Model file for the job. Use its own axes, mm. Face numbers are marked on the shaded views. A direction names the side the tool comes from. Coordinates: 2 decimals unless noted, no trailing zeros. Write each loop counter-clockwise with the first axis right and the second up, starting at its lowest first coordinate (ties: lowest second). Pieces come first, ordered by that corner, then holes. Notation, with made-up numbers: M 57.25,57 L 108.25,57 A12 ccw 108.25,80 Z; hole C 58.25,44.25 d2. An arc over 180 degrees is marked long. Put each result on its own line as item: value. Start each with the question number.
Q1. Cut at C-C (z = 17). Write the cut outline in (x, y), then the cut area to 3 significant figures.
Q2. Cut at B-B (y = -29). Write the cut outline in (x, z) (3 decimals), then the cut area to 3 significant figures.
Q3. Which spindle directions (+Z, -Z, +X, -X, +Y, -Y) get a long thin tool onto all of the face, cutting with end or side? Do the marked faces 1, 2, 3 and 4. Say none if no direction does.
Q4. Drop flat-ended pins along their axis: pin 1 (4 mm diameter, centred on y = -16, z = 12.5, fed in from -X); pin 2 (1 mm diameter, centred on y = -17.5, z = -7, fed in from -X); pin 3 (9.5 mm diameter, centred on x = 29, y = -5.5, fed in from -Z) (3 decimals). Give the stop position or say it passes through.
Q5. Drill centre lines: line 1 along Z through (x, y) = (6, -29); line 2 along Y through (x, z) = (36, 11); line 3 along Y through (x, z) = (38, 0.5). Where is each one in solid material? Low to high.
Q6. Cut at D-D (x = 3.5). Write the cut outline in (y, z).
Q7. Cut at A-A (x = 32.5). Write the cut outline in (y, z) (3 decimals).
Q8. Pull direction Y, two halves, no side cores. Call the marked faces 5, 6, 7 and 8: pulls with the +Y half, pulls with the -Y half, needs draft (parallel to the pull), parting line crosses it, or undercut.
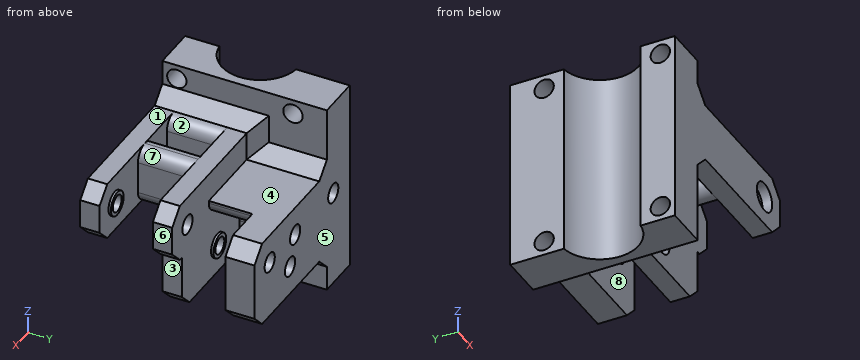
```python
from build123d import *

# Parameters (mm, degrees)
BOSS_EXTRUDE1_DEPTH      = 20
BOSS_EXTRUDE1_DEPTH_BACK = 20
SKETCH2_R                = 1.75
CUT_EXTRUDE1_DEPTH       = 59.72818744
SKETCH3_R                = 2
CUT_EXTRUDE2_DEPTH       = 7
CUT_EXTRUDE3_REACH       = 60.728
CUT_EXTRUDE4_REACH       = 54.783
CUT_EXTRUDE5_REACH       = 58.648
BOSS_EXTRUDE3_DEPTH      = 9
SKETCH10_W               = 5.38
SKETCH10_H               = 12
SKETCH10_W_2             = 5.81
BOSS_EXTRUDE4_DEPTH      = 11
FILLET1_R                = 2.69
FILLET2_R                = 2.69
FILLET3_R                = 2.69
CHAMFER1_SIZE            = 3
CUT_EXTRUDE8_REACH       = 51.774
SKETCH14_R               = 2
SKETCH16_R               = 2
CUT_EXTRUDE9_DEPTH       = 10
BOSS_EXTRUDE5_START      = 0.5
SKETCH17_R               = 2.5
SKETCH17_R_2             = 1.75
BOSS_EXTRUDE5_DEPTH      = 0.5
BOSS_EXTRUDE6_START      = 0.5
SKETCH18_R               = 2.5
SKETCH18_R_2             = 1.75
BOSS_EXTRUDE6_DEPTH      = 0.5
SKETCH20_R               = 3
CUT_EXTRUDE10_DEPTH      = 2
SKETCH21_R               = 3
CUT_EXTRUDE11_DEPTH      = 2
SKETCH11_R               = 2
CUT_EXTRUDE6_DEPTH       = 10
SKETCH12_W               = 1
SKETCH12_H               = 32
CUT_EXTRUDE7_DEPTH       = 67.426230512
BOSS_EXTRUDE7_DEPTH      = 4
BOSS_EXTRUDE8_START      = 2
SKETCH23_R               = 2
BOSS_EXTRUDE8_DEPTH      = 2


# Some blends are built 0.0001 mm under size
with BuildPart() as part:
    # Sketch1 → Boss-Extrude1 (new, two sides: drawn at the far end of the back side and taken through both)
    with BuildSketch(Plane.XY.offset(-BOSS_EXTRUDE1_DEPTH_BACK)):
        with BuildLine():
            Line((0, 0), (45, 0))
            Line((45, 0), (45, -4))
            Line((45, -4), (10, -4))
            Line((10, -4), (10, -13))
            Line((10, -13), (45, -13))
            Line((45, -13), (45, -17))
            Line((45, -17), (10, -17))
            Line((10, -17), (10, -28))
            Line((10, -28), (45, -28))
            Line((45, -28), (45, -32))
            Line((45, -32), (0, -32))
            Line((0, -32), (0, -28))
            Line((0, -28), (0, -25))
            ThreePointArc((0, -25), (8, -17), (0, -9))
            Line((0, -9), (0, -4))
            Line((0, -4), (0, 0))
        make_face()
    extrude(amount=BOSS_EXTRUDE1_DEPTH + BOSS_EXTRUDE1_DEPTH_BACK)

    # Sketch2 → Cut-Extrude1 (cut, through all)
    with BuildSketch(Plane(origin=(0, 0, 0), x_dir=(1, 0, 0), z_dir=(0, 1, 0))):
        with Locations(Location((24.5, 5.895, 0), (0, 0, 270))):
            Circle(SKETCH2_R)
        with Locations(Location((36.29, -5.895, 0), (0, 0, 270))):
            Circle(SKETCH2_R)
    extrude(amount=-CUT_EXTRUDE1_DEPTH, mode=Mode.SUBTRACT)

    # Sketch3 → Cut-Extrude2 (cut)
    with BuildSketch(Plane(origin=(0, 0, 0), x_dir=(1, 0, 0), z_dir=(0, 1, 0))):
        with Locations(Location((7.5, 0, 0), (0, 0, 270))):
            Circle(SKETCH3_R)
        with Locations(Location((22.5, 0, 0), (0, 0, 270))):
            Circle(SKETCH3_R)
        with Locations(Location((32.5, 0, 0), (0, 0, 270))):
            Circle(SKETCH3_R)
    extrude(amount=-CUT_EXTRUDE2_DEPTH, mode=Mode.SUBTRACT)

    # Sketch5 → Cut-Extrude3 (cut, up to next)
    with BuildSketch(Plane(origin=(0, 0, 0), x_dir=(1, 0, 0), z_dir=(0, 1, 0)), mode=Mode.PRIVATE) as cut_extrude3_sk1:
        Polygon((10, 20), (10, 11.895), (35.5, 11.895), (38.5, 8.895), (38.5, -3), (35.5, -6), (10, -6), (10, -20), (45, -20), (45, 20), align=None)
    cut_extrude3_tool1 = extrude(cut_extrude3_sk1.sketch, amount=-CUT_EXTRUDE3_REACH, mode=Mode.PRIVATE) & part.part
    add(cut_extrude3_tool1.solids().sort_by_distance((10.531507, 0, -15.9475))[0], mode=Mode.SUBTRACT)

    # Sketch6 → Cut-Extrude4 (cut, up to next)
    with BuildSketch(Plane(origin=(0, -13, 0), x_dir=(1, 0, 0), z_dir=(0, 1, 0)), mode=Mode.PRIVATE) as cut_extrude4_sk1:
        Polygon((45, 20), (10, 20), (10, 11.895), (35.5, 11.895), (38.5, 8.895), (38.5, 0.105), (39.29, 0.105), (42.29, -2.895), (42.29, -8.895), (39.29, -11.895), (10, -11.895), (10, -20), (45, -20), align=None)
    cut_extrude4_tool1 = extrude(cut_extrude4_sk1.sketch, amount=-CUT_EXTRUDE4_REACH, mode=Mode.PRIVATE) & part.part
    add(cut_extrude4_tool1.solids().sort_by_distance((27.5, -13, -19.468493))[0], mode=Mode.SUBTRACT)

    # Sketch7 → Cut-Extrude5 (cut, up to next)
    with BuildSketch(Plane(origin=(0, -28, 0), x_dir=(1, 0, 0), z_dir=(0, 1, 0)), mode=Mode.PRIVATE) as cut_extrude5_sk1:
        Polygon((10, -11.895), (39.29, -11.895), (42.29, -8.895), (42.29, -2.895), (39.29, 0.105), (10, 0.105), (10, 20), (45, 20), (45, -20), (10, -20), align=None)
    cut_extrude5_tool1 = extrude(cut_extrude5_sk1.sketch, amount=-CUT_EXTRUDE5_REACH, mode=Mode.PRIVATE) & part.part
    add(cut_extrude5_tool1.solids().sort_by_distance((28.13547, -28, -2.184137))[0], mode=Mode.SUBTRACT)

    # Sketch9 → Boss-Extrude3 (add)
    with BuildSketch(Plane(origin=(0, -13, 0), x_dir=(1, 0, 0), z_dir=(0, 1, 0))):
        with BuildLine():
            ThreePointArc((24.5, -2.795), (18.355242071, -0.249757929), (15.81, 5.895))
            Line((15.81, 5.895), (15.81, 11.895))
            Line((15.81, 11.895), (10, 11.895))
            Line((10, 11.895), (10, -6))
            Line((10, -6), (27.895, -6))
            Line((27.895, -6), (27.895, -2.795))
            Line((27.895, -2.795), (24.5, -2.795))
        make_face()
    extrude(amount=BOSS_EXTRUDE3_DEPTH)

    # Sketch10 → Boss-Extrude4 (add)
    with BuildSketch(Plane(origin=(0, -28, 0), x_dir=(1, 0, 0), z_dir=(0, 1, 0))):
        with Locations((24.5, -5.895)):
            Rectangle(SKETCH10_W, SKETCH10_H)
        with Locations((12.905, -5.895)):
            Rectangle(SKETCH10_W_2, SKETCH10_H)
    extrude(amount=BOSS_EXTRUDE4_DEPTH)

    # Fillet1
    # the kernel refuses this fillet: 2.69 mm, written as the material it adds along each edge
    # the kernel refuses this fillet: 2.69 mm, written as the material it takes off along each edge
    with BuildSketch(Plane(origin=(21.81, -28, -0.105), x_dir=(0, 0, 1), z_dir=(0, 1, 0))) as fillet1_2_piece_1:
        with BuildLine():
            CenterArc((FILLET1_R, FILLET1_R), FILLET1_R, 180, 90)
            Line((0, FILLET1_R), (0, 0))
            Line((0, 0), (FILLET1_R, 0))
        make_face()
    extrude(amount=11, mode=Mode.SUBTRACT)
    with BuildSketch(Plane(origin=(27.19, -28, -0.105), x_dir=(0, 0, 1), z_dir=(0, 1, 0))) as fillet1_2_piece_2:
        with BuildLine():
            CenterArc((FILLET1_R, -FILLET1_R), FILLET1_R, 90, 90)
            Line((0, -FILLET1_R), (0, 0))
            Line((0, 0), (FILLET1_R, 0))
        make_face()
    extrude(amount=11, mode=Mode.SUBTRACT)

    # Fillet2
    fillet2_edges = [part.edges().sort_by_distance(p)[0] for p in [
        (27.19, -22.5, 11.895),
        (21.81, -22.5, 11.895),
    ]]
    fillet(fillet2_edges, radius=FILLET2_R - 0.0001)  # a hair under: the kernel refuses the full size

    # Fillet3
    fillet3_edges = [part.edges().sort_by_distance(p)[0] for p in [
        (15.81, -8.5, -11.895),
        (27.895, -8.5, 2.795),
        (15.81, -22.5, -0.105),
        (15.81, -22.5, 11.895),
    ]]
    fillet(fillet3_edges, radius=FILLET3_R)

    # Chamfer1
    chamfer1_edges = [part.edges().sort_by_distance(p)[0] for p in [
        (10, -8.5, -11.895),
        (10, -6.5, 6),
        (10, -17, -6),
        (10, -22.5, 11.895),
        (10, -24.5, -0.105),
        (10, -13, 8.9475),
    ]]
    chamfer(chamfer1_edges, length=CHAMFER1_SIZE)

    # Sketch14 → Cut-Extrude8 (cut, up to next)
    with BuildSketch(Plane.XZ.offset(17), mode=Mode.PRIVATE) as cut_extrude8_sk1:
        with Locations(Location((36.29, 5.895, 0), (0, 0, 270))):
            Circle(SKETCH14_R)
    cut_extrude8_tool1 = extrude(cut_extrude8_sk1.sketch, amount=-CUT_EXTRUDE8_REACH, mode=Mode.PRIVATE) & part.part
    add(cut_extrude8_tool1.solids().sort_by_distance((36.29, -17, 5.895))[0], mode=Mode.SUBTRACT)

    # Sketch16 → Cut-Extrude9 (cut)
    with BuildSketch(Plane.XZ.offset(4)):
        with Locations((24.5, -5.895)):
            Circle(SKETCH16_R)
    extrude(amount=-CUT_EXTRUDE9_DEPTH, mode=Mode.SUBTRACT)

    # Sketch17 → Boss-Extrude5 (add)
    with BuildSketch(Plane(origin=(0, -13, 0), x_dir=(1, 0, 0), z_dir=(0, 1, 0)).offset(BOSS_EXTRUDE5_START)):
        with Locations(Location((24.5, 5.895, 0), (0, 0, 270))):
            Circle(SKETCH17_R)
        with Locations(Location((24.5, 5.895, 0), (0, 0, 270))):
            Circle(SKETCH17_R_2, mode=Mode.SUBTRACT)
    extrude(amount=-BOSS_EXTRUDE5_DEPTH)

    # Sketch18 → Boss-Extrude6 (add)
    with BuildSketch(Plane(origin=(0, -28, 0), x_dir=(1, 0, 0), z_dir=(0, 1, 0)).offset(BOSS_EXTRUDE6_START)):
        with Locations(Location((36.29, -5.895, 0), (0, 0, 270))):
            Circle(SKETCH18_R)
        with Locations(Location((36.29, -5.895, 0), (0, 0, 270))):
            Circle(SKETCH18_R_2, mode=Mode.SUBTRACT)
    extrude(amount=-BOSS_EXTRUDE6_DEPTH)

    # Sketch20 → Cut-Extrude10 (cut)
    with BuildSketch(Plane.XZ.offset(32)):
        with Locations(Location((36.29, 5.895, 0), (0, 0, 270))):
            Circle(SKETCH20_R)
    extrude(amount=-CUT_EXTRUDE10_DEPTH, mode=Mode.SUBTRACT)

    # Sketch21 → Cut-Extrude11 (cut)
    with BuildSketch(Plane.XZ.offset(17)):
        with Locations(Location((24.5, -5.895, 0), (0, 0, 270))):
            Circle(SKETCH21_R)
    extrude(amount=-CUT_EXTRUDE11_DEPTH, mode=Mode.SUBTRACT)

    # Sketch11 → Cut-Extrude6 (cut)
    with BuildSketch(Plane.ZY):
        with Locations(Location((17, -5, 0), (0, 0, 270))):
            Circle(SKETCH11_R)
        with Locations(Location((17, -29, 0), (0, 0, 270))):
            Circle(SKETCH11_R)
        with Locations(Location((-17, -29, 0), (0, 0, 270))):
            Circle(SKETCH11_R)
        with Locations(Location((-17, -5, 0), (0, 0, 270))):
            Circle(SKETCH11_R)
    extrude(amount=-CUT_EXTRUDE6_DEPTH, mode=Mode.SUBTRACT)

    # Sketch12 → Cut-Extrude7 (cut, through all)
    with BuildSketch(Plane.XY.offset(20)):
        with Locations((0.5, -16)):
            Rectangle(SKETCH12_W, SKETCH12_H)
    extrude(amount=-CUT_EXTRUDE7_DEPTH, mode=Mode.SUBTRACT)

    # Sketch22 → Boss-Extrude7 (add)
    with BuildSketch(Plane(origin=(0, 0, 0), x_dir=(1, 0, 0), z_dir=(0, 1, 0))):
        with BuildLine():
            Line((37.136593667, -4.363406333), (35.5, -6))
            Line((35.5, -6), (34.54315284, -6))
            ThreePointArc((34.54315284, -6), (35.356070776, -4.415041823), (37.136593667, -4.363406333))
        make_face()
    extrude(amount=-BOSS_EXTRUDE7_DEPTH)

    # Sketch23 → Boss-Extrude8 (add)
    with BuildSketch(Plane(origin=(0, 0, 0), x_dir=(1, 0, 0), z_dir=(0, 1, 0)).offset(BOSS_EXTRUDE8_START)):
        Polygon((35.5, 11.895), (13, 11.895), (10, 14.895), (10, 20), (1, 20), (1, -20), (10, -20), (10, -9), (13, -6), (35.5, -6), (38.5, -3), (38.5, 8.895), align=None)
        with Locations((24.5, 5.895)):
            Circle(SKETCH23_R, mode=Mode.SUBTRACT)
        with Locations(Location((32.5, 0, 0), (0, 0, 270))):
            Circle(SKETCH23_R, mode=Mode.SUBTRACT)
        with Locations(Location((22.5, 0, 0), (0, 0, 270))):
            Circle(SKETCH23_R, mode=Mode.SUBTRACT)
        with Locations(Location((7.5, 0, 0), (0, 0, 270))):
            Circle(SKETCH23_R, mode=Mode.SUBTRACT)
    extrude(amount=-BOSS_EXTRUDE8_DEPTH)


solid = part.part
```
Computed values:
1. outline: M 1,-32 L 10,-32 L 10,-31 L 1,-31 Z; M 1,-27 L 10,-27 L 10,-7 L 1,-7 L 1,-9.06 A8 cw 1,-24.94 Z; M 1,-3 L 10,-3 L 10,2 L 1,2 Z
1. area: 149 mm2
2. outline: M 1,-20 L 10,-20 L 10,-19 L 1,-19 Z; M 1,-15 L 10,-15 L 10,-3.105 L 13,-0.105 L 39.29,-0.105 L 42.29,2.895 L 42.29,8.895 L 39.29,11.895 L 13,11.895 L 10,14.895 L 10,15 L 1,15 Z; M 1,19 L 10,19 L 10,20 L 1,20 Z; hole C 36.29,5.895 d3.5
2. area: 666 mm2
3. face 1: +Z, +X, +Y, -Y
3. face 2: +Z
3. face 3: -Z, +X, +Y, -Y
3. face 4: +Z, +X, +Y
4. pin 1: x = 7.42
4. pin 2: x = 7.94
4. pin 3: z = -11.895
5. line 1: -20 to -19, -15 to 15, 19 to 20
5. line 2: -32 to -28, -17 to -13
5. line 3: -32 to -28, -17 to -13, -4 to 2
6. outline: M -32,-20 L -24.19,-20 L -24.19,20 L -32,20 Z; M -9.81,-20 L 2,-20 L 2,20 L -9.81,20 Z; hole C -29,-17 d4; hole C -29,17 d4; hole C -5,-17 d4; hole C -5,17 d4
7. outline: M -32,-0.105 L -28,-0.105 L -28,11.895 L -32,11.895 Z; M -17,-11.895 L -13,-11.895 L -13,11.895 L -17,11.895 Z; M -4,-11.895 L 2,-11.895 L 2,-2 L -4,-2 Z; M -4,2 L 2,2 L 2,6 L -4,6 Z
8. face 5: pulls with the +Y half
8. face 6: needs draft
8. face 7: undercut
8. face 8: undercut
